Source: CAD feature listing. Evaluate the final solid. Frame: model axes, mm. A direction names the side the tool comes from. Round coordinates to 2 decimals unless told otherwise and drop trailing zeros. Write each loop counter-clockwise with the first axis right and the second up, starting at its lowest first coordinate (ties: lowest second). Pieces come first, ordered by that corner, then holes. Notation, with made-up numbers: M -21.5,61.25 L 4.5,61.25 A17 ccw 4.5,83.25 Z; hole C 64.25,23 d6. An arc over 180 degrees is marked long. Answer in a Markdown table with one row per item.
from build123d import *

# Parameters (mm, degrees)
BASPROSKE_W           = 6
BASPROSKE_H           = 15
TOOTHCUT_DEPTH        = 23.045407685
TEETHCUTS_COUNT       = 28
TEETHCUTS_ANGLE       = 347.142857143
BORSKE_R              = 4
BORE_DEPTH            = 50.0000508
CROQUIS1_R            = 1.5
CORTAR_EXTRUIR1_DEPTH = 10


with BuildPart() as part:
    # BasProSke → Base-Revolve (revolve)
    with BuildSketch(Plane(origin=(0, 0, 0), x_dir=(1, 0, 0), z_dir=(0, 1, 0)), mode=Mode.PRIVATE) as base_revolve_sk:
        with Locations((3, 7.5)):
            Rectangle(BASPROSKE_W, BASPROSKE_H)
    revolve(base_revolve_sk.sketch.rotate(Axis((-10, 0, 0), (1, 0, 0)), 180), axis=Axis((-10, 0, 0), (1, 0, 0)))

    # TooCutSke → ToothCut (cut, through all)
    with BuildSketch(Plane(origin=(0, 0, 0), x_dir=(0, 0, -1), z_dir=(1, 0, 0))):
        with BuildLine():
            ThreePointArc((0.562705027, 12.736575837), (0, 12.749), (-0.562705027, 12.736575837))
            ThreePointArc((-0.562705027, 12.736575837), (-0.822951015, 13.892219122), (-1.32045988, 14.96726531))
            ThreePointArc((-1.32045988, 14.96726531), (0, 15.0254), (1.32045988, 14.96726531))
            ThreePointArc((1.32045988, 14.96726531), (0.822951015, 13.892219122), (0.562705027, 12.736575837))
        make_face()
    toothcut = extrude(amount=TOOTHCUT_DEPTH, mode=Mode.SUBTRACT)

    # TeethCuts: ToothCut ×28 about axis
    teethcuts_axis = Axis((-10, 0, 0), (1, 0, 0))
    for i in range(1, TEETHCUTS_COUNT):
        add(toothcut.rotate(teethcuts_axis, i * TEETHCUTS_ANGLE / (TEETHCUTS_COUNT - 1)), mode=Mode.SUBTRACT)

    # BorSke → Bore (cut, symmetric)
    with BuildSketch(Plane(origin=(0, 0, 0), x_dir=(0, 0, -1), z_dir=(1, 0, 0))):
        with Locations(Location((0, 0, 0), (0, 0, 180))):
            Circle(BORSKE_R)
    extrude(amount=BORE_DEPTH, both=True, mode=Mode.SUBTRACT)

    # Croquis1 → Cortar-Extruir1 (cut)
    with BuildSketch(Plane(origin=(6, 0, 0), x_dir=(0, 0, -1), z_dir=(1, 0, 0))):
        with Locations((-7.75, 0)):
            Circle(CROQUIS1_R)
        with Locations((7.75, 0)):
            Circle(CROQUIS1_R)
    extrude(amount=-CORTAR_EXTRUIR1_DEPTH, mode=Mode.SUBTRACT)


solid = part.part
Q1. Pull-direction query (Z, two-part tool) for faces 1 (the flat face through (0, 3, 4)), 2 (the cylindrical face through (2.96, -9.31, -10.35)), 3 (the cylindrical face through (2.96, 8.01, 11.35)); classes: pulls with the +Z half, pulls with the -Z half, needs draft (parallel to the pull), parting line crosses it, or undercut.
Solutions:
| item | result |
|---|---|
| face 1 | needs draft |
| face 2 | pulls with the -Z half |
| face 3 | undercut |
Q2. Section A-A (y = 0). Return loops of the section in (x, z), and give its area (3 significant figures).
Solutions:
| item | result |
|---|---|
| outline | M 0,-12.75 L 6,-12.75 L 6,-9.25 L 0,-9.25 Z; M 0,-6.25 L 6,-6.25 L 6,-4 L 0,-4 Z; M 0,4 L 6,4 L 6,6.25 L 0,6.25 Z; M 0,9.25 L 6,9.25 L 6,12.75 L 0,12.75 Z |
| area | 69.0 mm2 |
Q3. Access query for faces 4 (the cylindrical face through (2.96, 11.35, -8.01)), 5 (the cylindrical face through (2.958, -3.895, -13.363)), 6 (the cylindrical face through (2.958, -0.813, 13.863)), 7 (the cylindrical face through (2.96, 12.14, 6.75)). Directions: +Z, -Z, +X, -X, +Y, -Y. A direction counts if a zero-diameter tool reaches every point of the face in a straight line with its end or side. Return the directions, or none.
Solutions:
| item | result |
|---|---|
| face 4 | +X, -X |
| face 5 | -Z, +X, -X |
| face 6 | +Z, +X, -X |
| face 7 | +X, -X, +Y |
Q4. Material intervals for probe 1 along Z at (x, y) = (5.1, 7.75); probe 2 along Z at (x, y) = (1.5, -10.75); probe 3 along Y at (x, z) = (4.1, -11.5), sorted ascending.
Solutions:
| item | result |
|---|---|
| probe 1 | z = -12.84 to -10.75, -10.12 to 10.12, 10.75 to 12.84 |
| probe 2 | z = -10.46 to -10.05, -7.75 to 7.75, 10.05 to 10.46 |
| probe 3 | y = -8.06 to -6.21, -5.5 to 5.5, 6.21 to 8.06 |
Q5. Section B-B (z = 0). Return loops of the section in (x, y).
Solutions:
| item | result |
|---|---|
| outline | M 0,-12.75 L 6,-12.75 L 6,-4 L 0,-4 Z; M 0,4 L 6,4 L 6,12.75 L 0,12.75 Z |
Q6. Section D-D (y = -7). Return loops of the section in (x, z).
Solutions:
| item | result |
|---|---|
| outline | M 0,-12.38 L 6,-12.38 L 6,12.38 L 0,12.38 Z |
Q7. Contact query for flat-ended pins moving along their axis: pin 1 Ø2 at (x, y) = (3.5, -11.5) entering from -Z; pin 2 Ø3 at (x, y) = (2.5, -4) entering from -Z; pin 3 Ø2 at (x, y) = (1, -8.5) entering from -Z. Output: stop coordinate, or through.
Solutions:
| item | result |
|---|---|
| pin 1 | stops at z = -10.71 |
| pin 2 | stops at z = -14.28 |
| pin 3 | stops at z = -12.9 |
Q8. Section C-C (x = 1.55). State how many separate pieces and enclosed holes the cut face has, and give its area (3 significant figures).
Solutions:
| item | result |
|---|---|
| separate pieces | 1 |
| enclosed holes | 3 |
| area | 535 mm2 |
